Here's the drawing with two shaded views (mm, measured from the low corner). I have some questions. Round coordinates to 2 decimals unless told otherwise and drop trailing zeros. Order: outer loops, then holes, each group sorted by start corner. A loop starts at its lowest first (then second) coordinate and runs counter-clockwise, first axis right, second up. Notation, with made-up numbers: (34, 3) -> (60, 3) arc R32 ccw to (60, 31) -> close; hole circle Ø9 at (48, 33). An arc over 180 degrees is marked (long way). Put each result on its own line as item: value. Start each with the question number.
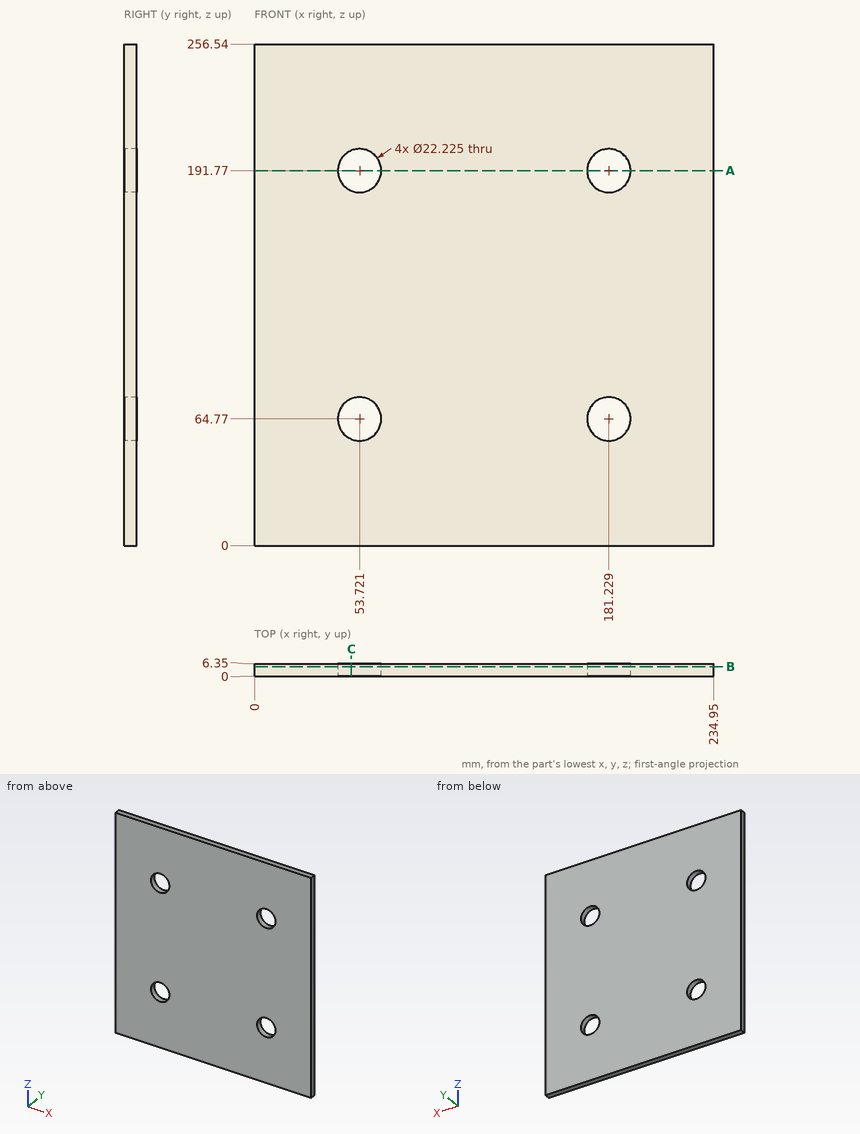
1. If we section it at C-C, the plane x = 49.5: Please give me the cut outline in (y, z), then the cut area to 3 significant figures.
2. If we section it at A-A, the plane z = 191.77: Please give me the cut outline in (x, y).
3. If we section it at B-B, the plane y = 4.75: Count the separate pieces of the cut face and the enclosed holes in it, then the cut area to 3 significant figures.
4. I need wall thicknesses on L1, parallel to X at y = 2, z = 181.5; L2, parallel to Z at x = 47, y = 1.75; L3, parallel to X at y = 2.5, z = 189. Which ranges of each line are inside material? Lowest first, please.
5. For pin 1 Ø20 at (x, z) = (53.721, 191.77) entering from +Y, with a flat end and sliding along its axis, tell me the tip position at first contact or that it passes through.
Results below:
1. outline: (0, 0) -> (6.35, 0) -> (6.35, 54.49) -> (0, 54.49) -> close; (0, 75.05) -> (6.35, 75.05) -> (6.35, 181.49) -> (0, 181.49) -> close; (0, 202.05) -> (6.35, 202.05) -> (6.35, 256.54) -> (0, 256.54) -> close
1. area: 1,370 mm2
2. outline: (0, 0) -> (42.61, 0) -> (42.61, 6.35) -> (0, 6.35) -> close; (64.83, 0) -> (170.12, 0) -> (170.12, 6.35) -> (64.83, 6.35) -> close; (192.34, 0) -> (234.95, 0) -> (234.95, 6.35) -> (192.34, 6.35) -> close
3. separate pieces: 1
3. enclosed holes: 4
3. area: 58,700 mm2
4. L1: 0 to 49.48, 57.97 to 176.98, 185.47 to 234.95
4. L2: 0 to 55.92, 73.62 to 182.92, 200.62 to 256.54
4. L3: 0 to 42.96, 64.48 to 170.47, 191.99 to 234.95
5. pin 1: through
